Work out the finished part from the listing and answer in its coordinate system (mm). Face numbers are marked on the shaded views. Give positions to 0.01 mm unless a question says otherwise; leave off trailing zeros. Order: outer loops, then holes, each group sorted by start corner. A loop starts at its lowest first (then second) coordinate and runs counter-clockwise, first axis right, second up. Notation, with made-up numbers: (-11, 37) - (37, 37) arc R16 cw to (37, 50) - close; hole circle Ø2 at (20.5, 89.5). An arc over 180 degrees is marked (long way). Put each result on its own line as item: value.
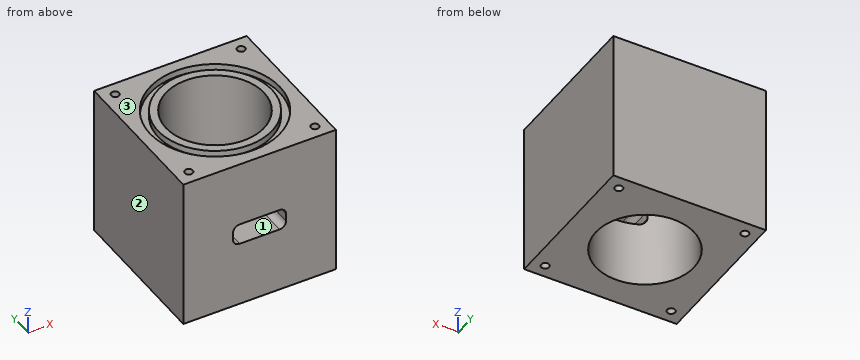
```python
from build123d import *

# Parameters (mm, degrees)
F0_W      = 152.4
F0_H      = 152.4
F1_DEPTH  = 152.4
F2_W      = 6.35
F2_H      = 152.4
F3_DEPTH  = 152.401
F4_W      = 6.35
F4_H      = 152.4
F5_DEPTH  = 146.051
F6_W      = 146.05
F6_H      = 6.35
F7_DEPTH  = 146.051
F8_R      = 3.81
F9_DEPTH  = 25.4
F8_R_2    = 62.23
F8_R_3    = 54.61
F10_DEPTH = 6.35
F8_R_4    = 46.99
F11_DEPTH = 146.051
F13_DEPTH = 50.8
F14_R     = 3.81
F15_DEPTH = 25.4


with BuildPart() as f1:
    # F0 (on Top) → F1 (new body)
    with BuildSketch(Plane.XY):
        Rectangle(F0_W, F0_H)
    extrude(amount=F1_DEPTH)

    # F2 (on face) → F3 (cut, through all)
    with BuildSketch(Plane.XZ.offset(76.2)):
        with Locations((73.025, 76.2)):
            Rectangle(F2_W, F2_H)
    extrude(amount=-F3_DEPTH, mode=Mode.SUBTRACT)

    # F4 (on face) → F5 (cut, through all)
    with BuildSketch(Plane.YZ.offset(69.85)):
        with Locations((73.025, 76.2)):
            Rectangle(F4_W, F4_H)
    extrude(amount=-F5_DEPTH, mode=Mode.SUBTRACT)

    # F6 (on face) → F7 (cut, through all)
    with BuildSketch(Plane.XZ.offset(76.2)):
        with Locations((-3.175, 149.225)):
            Rectangle(F6_W, F6_H)
    extrude(amount=-F7_DEPTH, mode=Mode.SUBTRACT)

    # F8 (on face) → F9 (cut)
    with BuildSketch(Plane.XY.offset(146.05)):
        with Locations((-63.5, 57.15)):
            Circle(F8_R)
        with Locations((57.15, 57.15)):
            Circle(F8_R)
        with Locations((57.15, -63.5)):
            Circle(F8_R)
        with Locations((-63.5, -63.5)):
            Circle(F8_R)
    extrude(amount=-F9_DEPTH, mode=Mode.SUBTRACT)

    # F8 (on face) → F10 (cut)
    with BuildSketch(Plane.XY.offset(146.05)):
        with Locations((-3.175, -3.175)):
            Circle(F8_R_2)
        with Locations((-3.175, -3.175)):
            Circle(F8_R_3, mode=Mode.SUBTRACT)
    extrude(amount=-F10_DEPTH, mode=Mode.SUBTRACT)

    # F8 (on face) → F11 (cut, through all)
    with BuildSketch(Plane.XY.offset(146.05)):
        with Locations((-3.175, -3.175)):
            Circle(F8_R_4)
    extrude(amount=-F11_DEPTH, mode=Mode.SUBTRACT)

    # F12 (on face) → F13 (cut)
    with BuildSketch(Plane.XZ.offset(76.2)):
        with BuildLine():
            ThreePointArc((22.225, 76.835), (20.3651280605, 81.3251280605), (15.875, 83.185))
            Line((15.875, 83.185), (-22.225, 83.185))
            ThreePointArc((-22.225, 83.185), (-26.7151280605, 81.3251280605), (-28.575, 76.835))
            Line((-28.575, 76.835), (-28.575, 69.215))
            ThreePointArc((-28.575, 69.215), (-26.7151280605, 64.7248719395), (-22.225, 62.865))
            Line((-22.225, 62.865), (15.875, 62.865))
            ThreePointArc((15.875, 62.865), (20.3651280605, 64.7248719395), (22.225, 69.215))
            Line((22.225, 69.215), (22.225, 76.835))
        make_face()
    extrude(amount=-F13_DEPTH, mode=Mode.SUBTRACT)

    # F14 (on face) → F15 (cut)
    with BuildSketch(Plane(origin=(0, 0, 0), x_dir=(1, 0, 0), z_dir=(0, 0, -1))):
        with Locations((-63.5, 63.5)):
            Circle(F14_R)
        with Locations((57.15, 63.5)):
            Circle(F14_R)
        with Locations((57.15, -57.15)):
            Circle(F14_R)
        with Locations((-63.5, -57.15)):
            Circle(F14_R)
    extrude(amount=-F15_DEPTH, mode=Mode.SUBTRACT)


solid = f1.part
```
(1) Section B-B, the plane y = -29 is taken. Write down the section's boundary in (x, z), then the cut area to 3 significant figures.
Geometry check:
outline: (-76.2, 0) - (-42.43, 0) - (-42.43, 146.05) - (-51.29, 146.05) - (-51.29, 139.7) - (-59.79, 139.7) - (-59.79, 146.05) - (-76.2, 146.05) - close; (36.08, 0) - (69.85, 0) - (69.85, 146.05) - (53.44, 146.05) - (53.44, 139.7) - (44.94, 139.7) - (44.94, 146.05) - (36.08, 146.05) - close
area: 9,760 mm²
(2) Straight lines are drawn through the part: line 1 (Y direction, x = 57, z = 13); line 2 (X direction, y = -63, z = 11). For each, find the intervals that lie inside material, in ascending order.
Geometry check:
line 1: y = -76.2 to -67.31, -59.69 to 53.34, 60.96 to 69.85
line 2: x = -76.2 to -67.28, -59.72 to 53.37, 60.93 to 69.85
(3) Given pin 1 (6 mm diameter, centred on x = 57.15, y = 57.15, fed in from +Z); pin 2 (2.5 mm diameter, centred on x = -64.5, y = -65, fed in from -Z), each flat-ended and moving along its own axis, determine where each tip first touches the part or whether it passes through.
Geometry check:
pin 1: stops at z = 120.65
pin 2: stops at z = 25.4
(4) Section C-C, the plane z = 56.5 is taken. Write down the section's boundary in (x, y) (3 decimals), then the cut area to 3 significant figures.
Geometry check:
outline: (-76.2, -76.2) - (69.85, -76.2) - (69.85, 69.85) - (-76.2, 69.85) - close; hole circle Ø93.98 at (-3.175, -3.175)
area: 14,400 mm²
(5) Section A-A, the plane x = 41 is taken. Write down the section's boundary in (y, z), then the cut area to 3 significant figures.
Geometry check:
outline: (-76.2, 0) - (-19.19, 0) - (-19.19, 146.05) - (-35.28, 146.05) - (-35.28, 139.7) - (-47.01, 139.7) - (-47.01, 146.05) - (-76.2, 146.05) - close; (12.84, 0) - (69.85, 0) - (69.85, 146.05) - (40.66, 146.05) - (40.66, 139.7) - (28.93, 139.7) - (28.93, 146.05) - (12.84, 146.05) - close
area: 16,500 mm²
(6) Determine the mould class of the marked faces 1, 2 and 3 for opening direction X: pulls with the +X half, pulls with the -X half, needs draft (parallel to the pull), parting line crosses it, or undercut.
Geometry check:
face 1: undercut
face 2: pulls with the -X half
face 3: needs draft
(7) Section D-D, the plane z = 128.5 is taken. Write down the section's boundary in (x, y) (3 decimals), then the cut area to 3 significant figures.
Geometry check:
outline: (-76.2, -76.2) - (69.85, -76.2) - (69.85, 69.85) - (-76.2, 69.85) - close; hole circle Ø7.62 at (-63.5, -63.5); hole circle Ø7.62 at (-63.5, 57.15); hole circle Ø93.98 at (-3.175, -3.175); hole circle Ø7.62 at (57.15, -63.5); hole circle Ø7.62 at (57.15, 57.15)
area: 14,200 mm²
